Print and shaded views of the part. All mm, measured from the part's lowest x, y and z. A direction names the side the tool comes from. Give positions to 0.01 mm unless a question says otherwise; leave off trailing zeros. Loops run counter-clockwise (first coordinate to the right, second up) from the corner with the lowest first, then second, coordinate; pieces in that order, holes last. Notation, with made-up numbers: M 0,-33 L 12,-33 A16 cw 12,-22 Z; hole C -24,20.5 d5. An arc over 180 degrees is marked long. Answer in a Markdown table with one row per item.
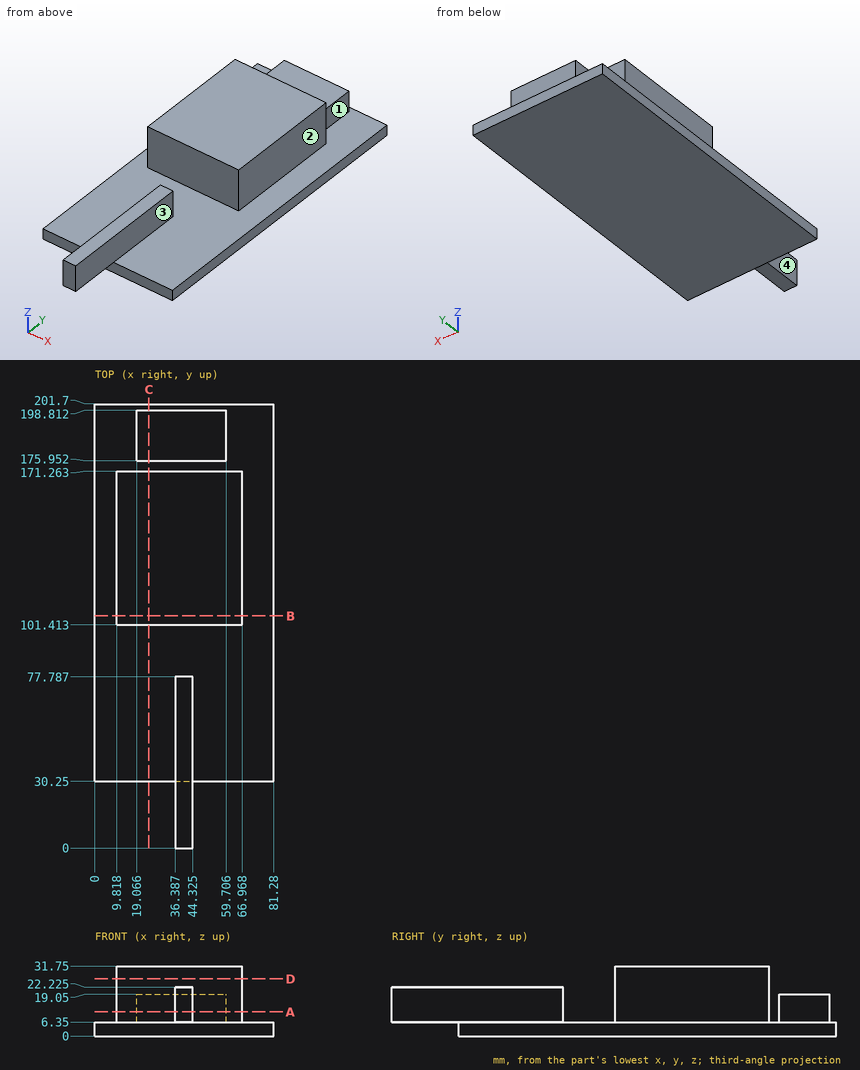
(1) Saw through at B-B, the plane y = 105.5. Give the cut face in (x, z), and give its area (3 significant figures).
Established:
| item | result |
|---|---|
| outline | M 0,0 L 81.28,0 L 81.28,6.35 L 66.97,6.35 L 66.97,31.75 L 9.82,31.75 L 9.82,6.35 L 0,6.35 Z |
| area | 1,970 mm2 |
(2) Saw through at A-A, the plane z = 11. Give the cut face in (x, y) (1 decimal).
Established:
| item | result |
|---|---|
| outline | M 9.8,101.4 L 67,101.4 L 67,171.3 L 9.8,171.3 Z; M 19.1,176 L 59.7,176 L 59.7,198.8 L 19.1,198.8 Z; M 36.4,0 L 44.3,0 L 44.3,77.8 L 36.4,77.8 Z |
(3) Saw through at C-C, the plane x = 24.5. Give the cut face in (y, z), and give its area (3 significant figures).
Established:
| item | result |
|---|---|
| outline | M 30.25,0 L 201.7,0 L 201.7,6.35 L 198.81,6.35 L 198.81,19.05 L 175.95,19.05 L 175.95,6.35 L 171.26,6.35 L 171.26,31.75 L 101.41,31.75 L 101.41,6.35 L 30.25,6.35 Z |
| area | 3,150 mm2 |
(4) Which spindle directions (+Z, -Z, +X, -X, +Y, -Y) get a long thin tool onto all of the face, cutting with end or side? Do the marked faces 1, 2, 3 and 4. Say none if no direction does.
Established:
| item | result |
|---|---|
| face 1 | +Z, +X, +Y |
| face 2 | +Z, +X, +Y, -Y |
| face 3 | +Z, +X, -Y |
| face 4 | +Z, -X, -Y |
(5) Saw through at D-D, the plane z = 26. Give the cut face in (x, y), and give its area (3 significant figures).
Established:
| item | result |
|---|---|
| outline | M 9.82,101.41 L 66.97,101.41 L 66.97,171.26 L 9.82,171.26 Z |
| area | 3,990 mm2 |
(6) Wall check: L1, parallel to Y at x = 34, z = 8.5; L2, parallel to Y at x = 17, z = 1.5; L3, parallel to X at y = 21, z = 7.5 (1 decimal). Give the ranges that are in metal, low to high.
Established:
| item | result |
|---|---|
| L1 | y = 101.41 to 171.26, 175.95 to 198.81 |
| L2 | y = 30.25 to 201.7 |
| L3 | x = 36.4 to 44.3 |
(7) Flat gauge pins, fed straight in: P1, Ø1, axis at y = 171, z = 7, coming from the -X side; P2, Ø4, axis at x = 51, z = 6, coming from the -Y side; P3, Ø5, axis at y = 25, z = 13.5, coming from the +X side (1 decimal). Where does each tip first touch, or does it go through?
Established:
| item | result |
|---|---|
| P1 | stops at x = 9.82 |
| P2 | stops at y = 30.25 |
| P3 | stops at x = 44.3 |
